The listing builds one solid part. Answer for the finished solid, in the listing's coordinates (mm). Coordinates: 2 decimals unless noted, no trailing zeros. Order: outer loops, then holes, each group sorted by start corner. A loop starts at its lowest first (then second) coordinate and runs counter-clockwise, first axis right, second up. Notation, with made-up numbers: (-6.5, -34) -> (45.5, -34) arc R10 ccw to (45.5, -30) -> close; hole circle Ø4 at (13.25, 18.5). An arc over 180 degrees is marked (long way). Return JSON: item names as keys, results as strings.
from build123d import *

# Parameters (mm, degrees)
SKETCH1_W           = 26.416
SKETCH1_H           = 32.004
BOSS_EXTRUDE1_DEPTH = 18.034
CHAMFER1_SIZE       = 12.54
CHAMFER2_SIZE       = 10
FILLET1_R           = 2.38


with BuildPart() as part:
    # Sketch1 → Boss-Extrude1 (new body)
    with BuildSketch(Plane(origin=(0, 0, 0), x_dir=(1, 0, 0), z_dir=(0, 1, 0))):
        with Locations((13.208, 16.002)):
            Rectangle(SKETCH1_W, SKETCH1_H)
    extrude(amount=BOSS_EXTRUDE1_DEPTH)

    # Chamfer1
    chamfer1_edges = [part.edges().sort_by_distance(p)[0] for p in [
        (13.208, 0, -32.004),
    ]]
    chamfer(chamfer1_edges, length=CHAMFER1_SIZE)

    # Chamfer2
    chamfer2_edges = [part.edges().sort_by_distance(p)[0] for p in [
        (13.208, 18.034, 0),
    ]]
    chamfer(chamfer2_edges, length=CHAMFER2_SIZE)

    # Fillet1
    fillet1_edges = [part.edges().sort_by_distance(p)[0] for p in [
        (13.208, 12.54, -32.004),
        (0, 0, -9.732),
        (0, 6.27, -25.734),
        (13.208, 0, -19.464),
        (26.416, 6.27, -25.734),
        (13.208, 18.034, -32.004),
        (26.416, 18.034, -21.002),
        (13.208, 18.034, -10),
        (26.416, 4.017, 0),
        (26.416, 13.034, -5),
        (0, 4.017, 0),
        (13.208, 8.034, 0),
        (0, 13.034, -5),
        (0, 18.034, -21.002),
        (26.416, 0, -9.732),
        (13.208, 0, 0),
        (0, 15.287, -32.004),
        (26.416, 15.287, -32.004),
    ]]
    fillet(fillet1_edges, radius=FILLET1_R)


solid = part.part
1. Consider line 1 (Y direction, x = 6.75, z = -25); line 2 (Z direction, x = 7.75, y = 11.75); line 3 (Y direction, x = 9.75, z = -3.5). Determine where each line is inside the solid, lowest interval first. Write a range as from..to.
Answer block:
{"line 1": "y = 5.54..18.03", "line 2": "z = -31.21..-3.72", "line 3": "y = 0..11.53"}
2. The part is cut by section A-A on x = 20.75. Give the vertices of the cut face in (y, z), and give its area (3 significant figures).
Answer block:
{"outline": "(0, -18.48) arc R2.38 ccw to (0.7, -20.16) -> (11.84, -31.31) arc R2.38 ccw to (13.53, -32) -> (15.65, -32) arc R2.38 ccw to (18.03, -29.62) -> (18.03, -10.99) arc R2.38 ccw to (17.34, -9.3) -> (8.73, -0.7) arc R2.38 ccw to (7.05, 0) -> (2.38, 0) arc R2.38 ccw to (0, -2.38) -> close", "area": "446 mm2"}
3. Each of these flat-tipped pins is pushed along its axis until it touches: pin 1 Ø8 at (x, y) = (18.5, 8) entering from +Z; pin 2 Ø5 at (x, y) = (19, 2.5) entering from -Z; pin 3 Ø6 at (y, z) = (2.5, -27) entering from +X; pin 4 Ø2 at (x, y) = (4.5, 14) entering from +Z. Where does it stop, or does it pass through?
Answer block:
{"pin 1": "stops at z = 0", "pin 2": "stops at z = -24.46", "pin 3": "passes through", "pin 4": "stops at z = -4.97"}
